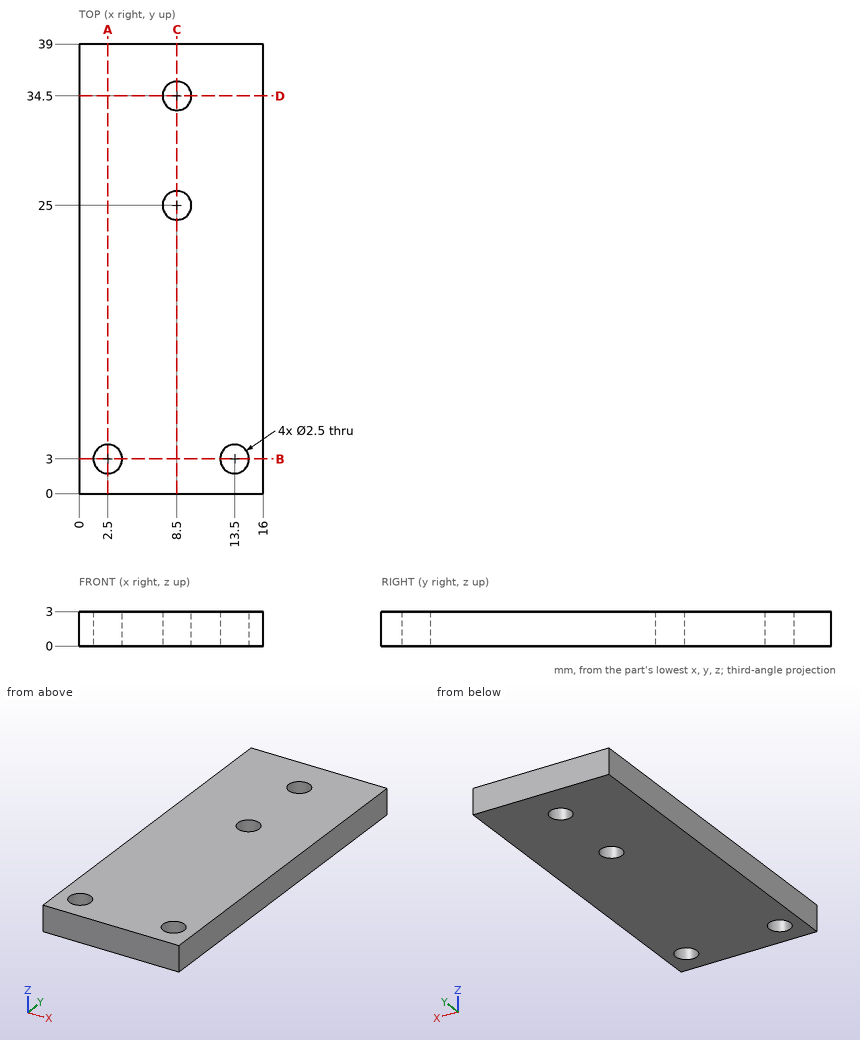
Verification items for this drawing (mm, ordinates from the low corner). Coordinates: 2 decimals unless noted, no trailing zeros. Loops run counter-clockwise (first coordinate to the right, second up) from the corner with the lowest first, then second, coordinate; pieces in that order, holes last. Notation, with made-up numbers: (-23, 33) - (9, 33) arc R18 cw to (9, 40) - close; hole circle Ø3 at (39, 14.5). An arc over 180 degrees is marked (long way). Answer as a JSON object with one key per item and string values.
(1) Cross-section at D-D, the plane y = 34.5. Record the boundary of the cut face in (x, z), then the cut area to 3 significant figures.
Response:
{"outline": "(0, 0) - (7.25, 0) - (7.25, 3) - (0, 3) - close; (9.75, 0) - (16, 0) - (16, 3) - (9.75, 3) - close", "area": "40.5 mm²"}
(2) Scan lines: line 1 along Y through (x, z) = (8.5, 1.95); line 2 along Y through (x, z) = (2.5, 1.25); line 3 along Y through (x, z) = (9.5, 2.85). Record each from-to range of solid material in increasing order.
Response:
{"line 1": "y = 0 to 23.75, 26.25 to 33.25, 35.75 to 39", "line 2": "y = 0 to 1.75, 4.25 to 39", "line 3": "y = 0 to 24.25, 25.75 to 33.75, 35.25 to 39"}
(3) Go/stop test with a flat-tipped pin: pin 1 Ø2 at (x, y) = (2.5, 3) entering from +Z. Record where the tip stops, or that it passes through.
Response:
{"pin 1": "passes through"}
(4) Cross-section at C-C, the plane x = 8.5. Record the boundary of the cut face in (y, z).
Response:
{"outline": "(0, 0) - (23.75, 0) - (23.75, 3) - (0, 3) - close; (26.25, 0) - (33.25, 0) - (33.25, 3) - (26.25, 3) - close; (35.75, 0) - (39, 0) - (39, 3) - (35.75, 3) - close"}
(5) Cross-section at B-B, the plane y = 3. Record the boundary of the cut face in (x, z), then the cut area to 3 significant figures.
Response:
{"outline": "(0, 0) - (1.25, 0) - (1.25, 3) - (0, 3) - close; (3.75, 0) - (12.25, 0) - (12.25, 3) - (3.75, 3) - close; (14.75, 0) - (16, 0) - (16, 3) - (14.75, 3) - close", "area": "33.0 mm²"}
(6) Cross-section at A-A, the plane x = 2.5. Record the boundary of the cut face in (y, z), then the cut area to 4 significant figures.
Response:
{"outline": "(0, 0) - (1.75, 0) - (1.75, 3) - (0, 3) - close; (4.25, 0) - (39, 0) - (39, 3) - (4.25, 3) - close", "area": "109.5 mm²"}
